Can you work these out from the model? Positions are in its coordinate system, mm. A direction names the side the tool comes from. Give positions to 0.01 mm unless a question says otherwise; leave off trailing zeros. Loops run counter-clockwise (first coordinate to the right, second up) from the corner with the lowest first, then second, coordinate; pieces in that order, holes last.
from build123d import *

# Parameters (mm, degrees)
BOSS_EXTRUDE1_DEPTH = 20
SKETCH2_R           = 3
CUT_EXTRUDE2_DEPTH  = 39
FILLET1_R           = 0.5
SKETCH4_R           = 5.872078672
BOSS_EXTRUDE2_DEPTH = 1
SKETCH5_R           = 3.732814836
BOSS_EXTRUDE3_DEPTH = 2
SKETCH8_R           = 1.5
BOSS_EXTRUDE4_DEPTH = 2


with BuildPart() as part:
    # Sketch1 → Boss-Extrude1 (new body)
    with BuildSketch(Plane.XY):
        Polygon((-29, 19), (29, 19), (29, 15.862733035), (20.5, 15.862733035), (20.5, -19), (-20.5, -19), (-20.5, 15.862733035), (-29, 15.862733035), align=None)
    extrude(amount=-BOSS_EXTRUDE1_DEPTH)

    # Sketch2 → Cut-Extrude2 (cut, through all)
    with BuildSketch(Plane(origin=(0, 19, 0), x_dir=(1, 0, 0), z_dir=(0, 1, 0))):
        with Locations((26.5, 5)):
            Circle(SKETCH2_R)
        with Locations((26.5, 15)):
            Circle(SKETCH2_R)
        with Locations((-26.5, 5)):
            Circle(SKETCH2_R)
        with Locations((-26.5, 15)):
            Circle(SKETCH2_R)
    extrude(amount=-CUT_EXTRUDE2_DEPTH, mode=Mode.SUBTRACT)

    # Fillet1
    fillet1_edges = [part.edges().sort_by_distance(p)[0] for p in [
        (29, 17.431366518, -3.341687605),
        (29, 17.431366518, -6.658312395),
        (29, 17.431366518, -13.341687605),
        (29, 17.431366518, -16.658312395),
        (-29, 17.431366518, -3.341687605),
        (-29, 17.431366518, -6.658312395),
        (-29, 17.431366518, -13.341687605),
        (-29, 17.431366518, -16.658312395),
    ]]
    fillet(fillet1_edges, radius=FILLET1_R)

    # Sketch4 → Boss-Extrude2 (add)
    with BuildSketch(Plane(origin=(0, 19, 0), x_dir=(1, 0, 0), z_dir=(0, 1, 0))):
        with Locations((-15.375793184, 10)):
            Circle(SKETCH4_R)
    extrude(amount=BOSS_EXTRUDE2_DEPTH)

    # Sketch5 → Boss-Extrude3 (add)
    with BuildSketch(Plane(origin=(0, 20, 0), x_dir=(1, 0, 0), z_dir=(0, 1, 0))):
        with Locations((-15.375793184, 10)):
            Circle(SKETCH5_R)
    extrude(amount=BOSS_EXTRUDE3_DEPTH)

    # Sketch8 → Boss-Extrude4 (add)
    with BuildSketch(Plane(origin=(0, 22, 0), x_dir=(1, 0, 0), z_dir=(0, 1, 0))):
        with Locations((-15.375793184, 10)):
            Circle(SKETCH8_R)
    extrude(amount=BOSS_EXTRUDE4_DEPTH)


solid = part.part
(1) Suppose I cut it at B-B on z = -10. List the corners of the cut face in (x, y) for me, plus the area to 3 significant figures.
Returned:
outline: (-29, 15.86) - (-20.5, 15.86) - (-20.5, -19) - (20.5, -19) - (20.5, 15.86) - (29, 15.86) - (29, 19) - (-9.5, 19) - (-9.5, 20) - (-11.64, 20) - (-11.64, 22) - (-13.88, 22) - (-13.88, 24) - (-16.88, 24) - (-16.88, 22) - (-19.11, 22) - (-19.11, 20) - (-21.25, 20) - (-21.25, 19) - (-29, 19) - close
area: 1,640 mm2
(2) Suppose I cut it at A-A on x = -26.5. List the corners of the cut face in (y, z) for me.
Returned:
outline: (15.86, -20) - (19, -20) - (19, -18) - (15.86, -18) - close; (15.86, -12) - (19, -12) - (19, -8) - (15.86, -8) - close; (15.86, -2) - (19, -2) - (19, 0) - (15.86, 0) - close
(3) Will these pins go through, and if not, where does the flat tip stop? P1, Ø4, axis at x = 23.5, z = -7, coming from the -Y side; P2, Ø1, axis at y = -11, z = -16.5, coming from the -X side; P3, Ø9.5, axis at x = 26.5, z = -5, coming from the +Y side.
Returned:
P1: stops at y = 15.86
P2: stops at x = -20.5
P3: stops at y = 19
(4) Suppose I cut it at D-D on x = 4.5. List the corners of the cut face in (y, z) for me.
Returned:
outline: (-19, -20) - (19, -20) - (19, 0) - (-19, 0) - close
(5) Suppose I cut it at C-C on y = 18. List the corners of the cut face in (x, z) for me, plus the area to 3 significant figures.
Returned:
outline: (-29, -20) - (29, -20) - (29, -17.87) arc R0.5 ccw to (28.21, -17.46) arc R3 cw (long way) to (28.21, -12.54) arc R0.5 ccw to (29, -12.13) - (29, -7.87) arc R0.5 ccw to (28.21, -7.46) arc R3 cw (long way) to (28.21, -2.54) arc R0.5 ccw to (29, -2.13) - (29, 0) - (-29, 0) - (-29, -2.13) arc R0.5 ccw to (-28.21, -2.54) arc R3 cw (long way) to (-28.21, -7.46) arc R0.5 ccw to (-29, -7.87) - (-29, -12.13) arc R0.5 ccw to (-28.21, -12.54) arc R3 cw (long way) to (-28.21, -17.46) arc R0.5 ccw to (-29, -17.87) - close
area: 1,050 mm2
(6) Which directions (+Z, -Z, +X, -X, +Y, -Y) give clear straight access to the entire face, cutting with the end or side of a thin tool? Please do faces 5 (the flat face through (-24, 15.863, -10)), 6 (the flat face through (20.5, -1, -10)), 7 (the flat face through (-15, 22, -8)), 8 (the flat face through (-29, 17, -10)).
Returned:
face 5: +Z, -Z, -X, -Y
face 6: +Z, -Z, +X, -Y
face 7: +Y
face 8: +Z, -Z, -X, +Y, -Y
(7) Please list where these lines run through material, in increasing order: probe 1 along Z at (x, y) = (-26.5, 16.7); probe 2 along X at (y, z) = (-2, -9); probe 3 along Y at (x, z) = (-2, -4.5).
Returned:
probe 1: z = -20 to -18, -12 to -8, -2 to 0
probe 2: x = -20.5 to 20.5
probe 3: y = -19 to 19
(8) Thinking about a two-plate mould opening in X: for faces 1 (the flat face through (-29, 17, -1)), 2 (the cylindrical face through (23.5, 17.5, -5.1)), 3 (the cylindrical face through (23.5, 17.5, -15.1)), 4 (the cylindrical face through (-14, 23, -9.4)), which applies, pulls with the +X half, pulls with the -X half, needs draft (parallel to the pull), parting line crosses it, or undercut?
Returned:
face 1: pulls with the -X half
face 2: undercut
face 3: undercut
face 4: parting line crosses it
